Check sheet for the modelled part. Datum: model origin and axes. Units: mm. Face numbers are marked on the shaded views. A direction names the side the tool comes from. Round coordinates to 2 decimals unless told otherwise and drop trailing zeros. Write each loop counter-clockwise with the first axis right and the second up, starting at its lowest first coordinate (ties: lowest second). Pieces come first, ordered by that corner, then holes. Notation, with made-up numbers: M 66,33 L 90,33 A28 ccw 90,70 Z; hole C -26.75,53 d6. An arc over 180 degrees is marked long. One line per item, written item: value.
from build123d import *

# Parameters (mm, degrees)
F0_W      = 76.2
F0_H      = 63.5
F0_W_2    = 31.75
F0_H_2    = 25.4
F1_DEPTH  = 25.4
F2_W      = 31.75
F2_H      = 25.4
F3_DEPTH  = 31.75
F6_DEPTH  = 6.35
F7_W      = 4.2333333333
F7_H      = 19.05
F8_DEPTH  = 31.751
F9_R      = 3.175
F10_DEPTH = 44.451


with BuildPart() as f1:
    # F0 (on Front) → F1 (new body)
    with BuildSketch(Plane.XZ):
        Rectangle(F0_W, F0_H)
        with Locations((19.05, 15.875)):
            Rectangle(F0_W_2, F0_H_2, mode=Mode.SUBTRACT)
    extrude(amount=F1_DEPTH)

    # F2 (on face) → F3 (join)
    with BuildSketch(Plane(origin=(0, 0, 0), x_dir=(-1, 0, 0), z_dir=(0, 1, 0))):
        with Locations((-19.05, 15.875)):
            Rectangle(F2_W, F2_H)
    extrude(amount=-F3_DEPTH)

    # F5 (on offset) → F6 (join, symmetric)
    with BuildSketch(Plane(origin=(0, 0, 0), x_dir=(0, -1, 0), z_dir=(-1, 0, 0))):
        with BuildLine():
            Line((6.35, -31.75), (6.35, -44.45))
            ThreePointArc((6.35, -44.45), (12.7, -50.8), (19.05, -44.45))
            Line((19.05, -44.45), (19.05, -31.75))
            Line((19.05, -31.75), (6.35, -31.75))
        make_face()
    extrude(amount=F6_DEPTH, both=True)

    # F7 (on Front) → F8 (cut, through all)
    with BuildSketch(Plane.XZ):
        with Locations((0, -41.275)):
            Rectangle(F7_W, F7_H)
    extrude(amount=F8_DEPTH, mode=Mode.SUBTRACT)

    # F9 (on face) → F10 (cut, through all)
    with BuildSketch(Plane.YZ.offset(6.35)):
        with Locations((-12.7, -44.45)):
            Circle(F9_R)
    extrude(amount=-F10_DEPTH, mode=Mode.SUBTRACT)


solid = f1.part
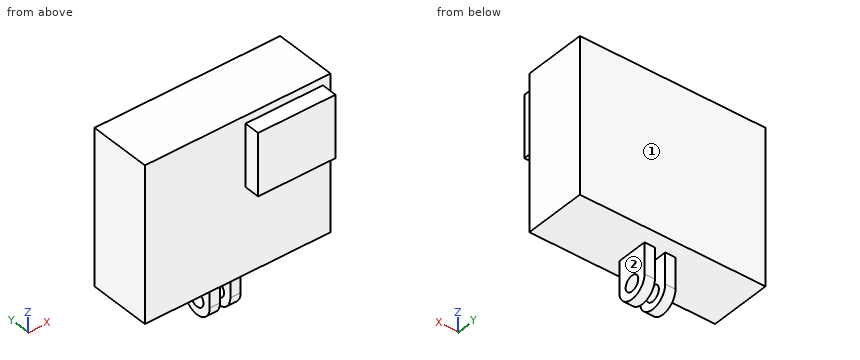
Q1. Sectioned sample at D-D on y = -22.5. Enter the section's corners in (x, z), and give its area (3 significant figures).
Completed:
outline: M -38.1,-31.75 L 38.1,-31.75 L 38.1,31.75 L -38.1,31.75 Z
area: 4,840 mm^2
Q2. Scan lines: line 1 (Z direction, x = 3.4, y = -12.7) (3 decimals); line 2 (Y direction, x = 18, z = -26.5); line 3 (Z direction, x = 17, y = -1.5). Record each from-to range of solid material in increasing order. Write a range as [from, to].
Completed:
line 1: [-50.8, -47.625], [-41.275, 31.75]
line 2: [-25.4, 0]
line 3: [-31.75, 31.75]
Q3. Access from +Z, -Z, +X, -X, +Y, -Y to the whole of each face (thin tool, end or side, straight path). Record for the marked faces 1 and 2.
Completed:
face 1: +Z, -Z, +X, -X, +Y
face 2: -Z, +X, +Y, -Y
Q4. Sectioned sample at B-B on z = 18. Enter the section's corners in (x, y) (3 decimals), and give its area (3 significant figures).
Completed:
outline: M -38.1,-25.4 L 3.175,-25.4 L 3.175,-31.75 L 34.925,-31.75 L 34.925,-25.4 L 38.1,-25.4 L 38.1,0 L -38.1,0 Z
area: 2,140 mm^2
Q5. Depth check by flat-ended pin: P1, Ø8.5, axis at y = -12.7, z = -44.45, coming from the -X side; P2, Ø3, axis at x = 21.5, y = -29, coming from the -Z side (3 decimals); P3, Ø6.5, axis at y = -12, z = -39.5, coming from the +X side; P4, Ø5.5, axis at y = -12.7, z = -44.45, coming from the +X side. Enter the tip coordinate at first touch or a pass-through.
Completed:
P1: x = -6.35
P2: z = 3.175
P3: x = 6.35
P4: through
Q6. Sectioned sample at C-C on x = 8.5. Enter the section's corners in (y, z) (3 decimals).
Completed:
outline: M -31.75,3.175 L -25.4,3.175 L -25.4,-31.75 L 0,-31.75 L 0,31.75 L -25.4,31.75 L -25.4,28.575 L -31.75,28.575 Z
Q7. Sectioned sample at A-A on y = -12.7. Enter the section's corners in (x, z) (3 decimals), and give its area (3 significant figures).
Completed:
outline: M -38.1,-31.75 L -6.35,-31.75 L -6.35,-41.275 L -2.117,-41.275 L -2.117,-31.75 L 2.117,-31.75 L 2.117,-41.275 L 6.35,-41.275 L 6.35,-31.75 L 38.1,-31.75 L 38.1,31.75 L -38.1,31.75 Z; M -6.35,-50.8 L -2.117,-50.8 L -2.117,-47.625 L -6.35,-47.625 Z; M 2.117,-50.8 L 6.35,-50.8 L 6.35,-47.625 L 2.117,-47.625 Z
area: 4,950 mm^2
